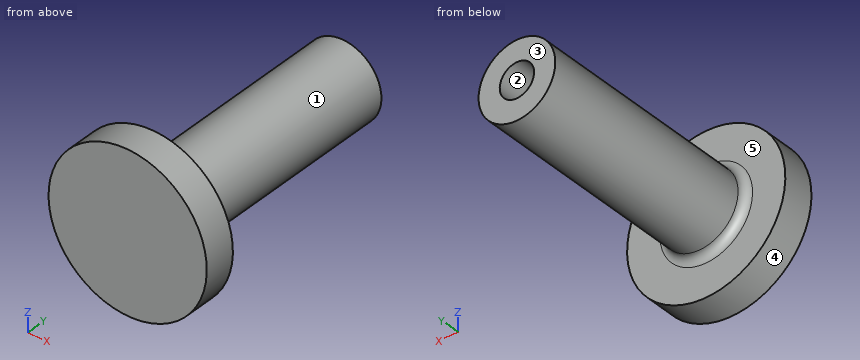
```python
from build123d import *

# Parameters (mm, degrees)
SKETCH1_R           = 9.9
SKETCH1_R_2         = 4.8
SKETCH1_R_3         = 2.15
BOSS_EXTRUDE1_DEPTH = 4
BOSS_EXTRUDE2_START = 4
SKETCH1_3_R         = 4.8
SKETCH1_3_R_2       = 2.15
BOSS_EXTRUDE2_DEPTH = 29
CUT_EXTRUDE1_START  = 33
SKETCH1_4_R         = 2.15
CUT_EXTRUDE1_DEPTH  = 8
FILLET1_R           = 1


with BuildPart() as part:
    # Sketch1 → Boss-Extrude1 (new body)
    with BuildSketch(Plane(origin=(0, 0, 0), x_dir=(1, 0, 0), z_dir=(0, 1, 0))):
        with Locations(Location((0, 0, 0), (0, 0, 270))):
            Circle(SKETCH1_R)
        Circle(SKETCH1_R_2, mode=Mode.SUBTRACT)
        Circle(SKETCH1_R_2)
        Circle(SKETCH1_R_3, mode=Mode.SUBTRACT)
        Circle(SKETCH1_R_3)
    extrude(amount=BOSS_EXTRUDE1_DEPTH)

    # Sketch1<3> → Boss-Extrude2 (add)
    with BuildSketch(Plane(origin=(0, 0, 0), x_dir=(1, 0, 0), z_dir=(0, 1, 0)).offset(BOSS_EXTRUDE2_START)):
        with Locations(Location((0, 0, 0), (0, 0, 90))):
            Circle(SKETCH1_3_R)
        Circle(SKETCH1_3_R_2, mode=Mode.SUBTRACT)
        Circle(SKETCH1_3_R_2)
    extrude(amount=BOSS_EXTRUDE2_DEPTH)

    # Sketch1<4> → Cut-Extrude1 (cut)
    with BuildSketch(Plane(origin=(0, 0, 0), x_dir=(1, 0, 0), z_dir=(0, 1, 0)).offset(CUT_EXTRUDE1_START)):
        with Locations(Location((0, 0, 0), (0, 0, 270))):
            Circle(SKETCH1_4_R)
    extrude(amount=-CUT_EXTRUDE1_DEPTH, mode=Mode.SUBTRACT)

    # Fillet1
    fillet1_edges = [part.edges().sort_by_distance(p)[0] for p in [
        (0, 4, 4.8),
    ]]
    fillet(fillet1_edges, radius=FILLET1_R)


solid = part.part
```
Verification items for the finished model (mm, model axes). Face numbers are marked on the shaded views. A direction names the side the tool comes from. Give positions to 0.01 mm unless a question says otherwise; leave off trailing zeros. Loops run counter-clockwise (first coordinate to the right, second up) from the corner with the lowest first, then second, coordinate; pieces in that order, holes last. Notation, with made-up numbers: M 20.25,14.5 L 52.25,14.5 A18 ccw 52.25,46.5 Z; hole C 71.5,4.5 d3. An arc over 180 degrees is marked long. Return JSON: item names as keys, results as strings.
1) Section check C-C, the plane z = 0. Enter the section's corners in (x, y).
Findings:
{"outline": "M -9.9,0 L 9.9,0 L 9.9,4 L 5.8,4 A1 cw 4.8,5 L 4.8,33 L 2.15,33 L 2.15,25 L -2.15,25 L -2.15,33 L -4.8,33 L -4.8,5 A1 cw -5.8,4 L -9.9,4 Z"}
2) Tool access check on the marked faces 4 and 5. Record the directions out of +Z, -Z, +X, -X, +Y, -Y that give a thin tool (end or side, any length) a straight path to the whole face; none if there is none.
Findings:
{"face 4": "+Y, -Y", "face 5": "+Y"}
3) Material ranges on L1, parallel to X at y = 30.5, z = 0; L2, parallel to Y at x = -7.5, z = -4.5; L3, parallel to Z at x = 3, y = 5.5, recorded low to high. Write a range as [from, to].
Findings:
{"L1": "x = [-4.8, -2.15], [2.15, 4.8]", "L2": "y = [0, 4]", "L3": "z = [-3.75, 3.75]"}
4) Section check A-A, the plane y = 30. Enter the section's corners in (x, z), and give its area (3 significant figures).
Findings:
{"outline": "C 0,0 d9.6; hole C 0,0 d4.3", "area": "57.9 mm2"}
5) Gauge pin test, flat ends, axial feed: P1, Ø2, axis at y = 14.5, z = 1.5, coming from the +X side; P2, Ø1.5, axis at x = 6, y = 27, coming from the -Z side; P3, Ø2, axis at x = -5, y = 4, coming from the -Z side. Record the tip position at first contact, or that the pin passes through.
Findings:
{"P1": "stops at x = 4.77", "P2": "passes through", "P3": "stops at z = -9.06"}
6) Section check B-B, the plane x = 0. Enter the section's corners in (y, z).
Findings:
{"outline": "M 0,-9.9 L 4,-9.9 L 4,-5.8 A1 cw 5,-4.8 L 33,-4.8 L 33,-2.15 L 25,-2.15 L 25,2.15 L 33,2.15 L 33,4.8 L 5,4.8 A1 cw 4,5.8 L 4,9.9 L 0,9.9 Z"}
7) Mould release check, pull along Z, two halves, no side actions. Record for the marked faces 1, 2 and 3: released by +Z, released by -Z, zero draft, split by the parting line, or undercut.
Findings:
{"face 1": "split by the parting line", "face 2": "undercut", "face 3": "zero draft"}
8) Section check D-D, the plane y = 22.5. Enter the section's corners in (x, z).
Findings:
{"outline": "C 0,0 d9.6"}
